from build123d import *

# Parameters (mm, degrees)
SKETCH2_R            = 7.9375
PISTONE_BASE_DEPTH   = 38.1
SKETCH3_R            = 6.35
DRILL_HOLE_1_DEPTH   = 19.05
TOP_WHOLE_DEPTH      = 40.71923731
TOP_WHOLE_DEPTH_BACK = 40.71923731
SKETCH6_R            = 1.3589


with BuildPart() as part:
    # Sketch2 → Pistone Base (new body)
    with BuildSketch(Plane(origin=(0, 0, 0), x_dir=(1, 0, 0), z_dir=(0, 1, 0))):
        with Locations(Location((0, 0, 0), (0, 0, 90))):
            Circle(SKETCH2_R)
    extrude(amount=PISTONE_BASE_DEPTH)

    # Sketch3 → Drill Hole 1 (cut)
    with BuildSketch(Plane(origin=(0, 38.1, 0), x_dir=(1, 0, 0), z_dir=(0, 1, 0))):
        with Locations(Location((0, 0, 0), (0, 0, 270))):
            Circle(SKETCH3_R)
    extrude(amount=-DRILL_HOLE_1_DEPTH, mode=Mode.SUBTRACT)

    # Sketch6 → Top Whole (cut, two sides: drawn at the far end of the back side and taken through both)
    with BuildSketch(Plane(origin=(0, 0, 0), x_dir=(0, 0, -1), z_dir=(1, 0, 0)).offset(-TOP_WHOLE_DEPTH_BACK)):
        with Locations((-0.502050886, 33.3248)):
            Circle(SKETCH6_R)
    extrude(amount=TOP_WHOLE_DEPTH + TOP_WHOLE_DEPTH_BACK, mode=Mode.SUBTRACT)


solid = part.part
Could you check a few things on this model? Use its own coordinates, in mm. A direction names the side the tool comes from. Give positions to 0.01 mm unless a question says otherwise; leave off trailing zeros. Order: outer loops, then holes, each group sorted by start corner. A loop starts at its lowest first (then second) coordinate and runs counter-clockwise, first axis right, second up.
1. For pin 1 (4 mm diameter, centred on x = -1, z = 2.5, fed in from +Y); pin 2 (4 mm diameter, centred on x = 5.5, y = 18, fed in from -Z); pin 3 (4 mm diameter, centred on x = 5, z = -3.5, fed in from -Y); pin 4 (2 mm diameter, centred on y = 28, z = 1.5, fed in from -X), each with a flat end and sliding along its axis, tell me the tip position at first contact or that it passes through.
Answers below:
pin 1: stops at y = 19.05
pin 2: stops at z = -7.12
pin 3: stops at y = 0
pin 4: stops at x = -7.92
2. Suppose I cut it at A-A (x = 0). Write out the boundary of the cut face in (y, z), plus the area to 3 significant figures.
Answers below:
outline: (0, -7.94) - (38.1, -7.94) - (38.1, -6.35) - (19.05, -6.35) - (19.05, 6.35) - (38.1, 6.35) - (38.1, 7.94) - (0, 7.94) - close
area: 363 mm2
3. I need wall thicknesses on L1, parallel to X at y = 25.5, z = 0; L2, parallel to Y at x = 1.75, z = -4.5; L3, parallel to Z at x = -5.75, y = 31. Which ranges of each line are inside material? Lowest first, please.
Answers below:
L1: x = -7.94 to -6.35, 6.35 to 7.94
L2: y = 0 to 19.05
L3: z = -5.47 to -2.69, 2.69 to 5.47
4. Which directions (+Z, -Z, +X, -X, +Y, -Y) give clear straight access to the entire face, cutting with the end or side of a thin tool? Please do faces 1 (the flat face through (-7, 38.1, 0)), 2 (the cylindrical face through (-3.86, 28.71, -5.04)).
Answers below:
face 1: +Z, -Z, +X, -X, +Y
face 2: +Y
5. Suppose I cut it at C-C (y = 6.5). Write out the boundary of the cut face in (x, z) (1 decimal).
Answers below:
outline: circle Ø15.9 at (0, 0)
6. Suppose I cut it at D-D (x = 2.5). Write out the boundary of the cut face in (y, z).
Answers below:
outline: (0, -7.53) - (38.1, -7.53) - (38.1, -5.84) - (19.05, -5.84) - (19.05, 5.84) - (38.1, 5.84) - (38.1, 7.53) - (0, 7.53) - close
7. Suppose I cut it at B-B (z = 0). Write out the boundary of the cut face in (x, y), plus the area to 3 significant figures.
Answers below:
outline: (-7.94, 0) - (7.94, 0) - (7.94, 32.06) - (6.35, 32.06) - (6.35, 19.05) - (-6.35, 19.05) - (-6.35, 32.06) - (-7.94, 32.06) - close; (-7.94, 34.59) - (-6.35, 34.59) - (-6.35, 38.1) - (-7.94, 38.1) - close; (6.35, 34.59) - (7.94, 34.59) - (7.94, 38.1) - (6.35, 38.1) - close
area: 355 mm2
8. Thinking about a two-plate mould opening in X: for faces 3 (the cylindrical face through (7.75, 18.78, 1.72)), 4 (the flat face through (0, 19.05, 0)), 5 (the cylindrical face through (6.99, 32.8, -0.75)), which applies, +X half, -X half, draft (parallel to the pull), parting line (faces both ways), or undercut?
Answers below:
face 3: parting line
face 4: undercut
face 5: draft
